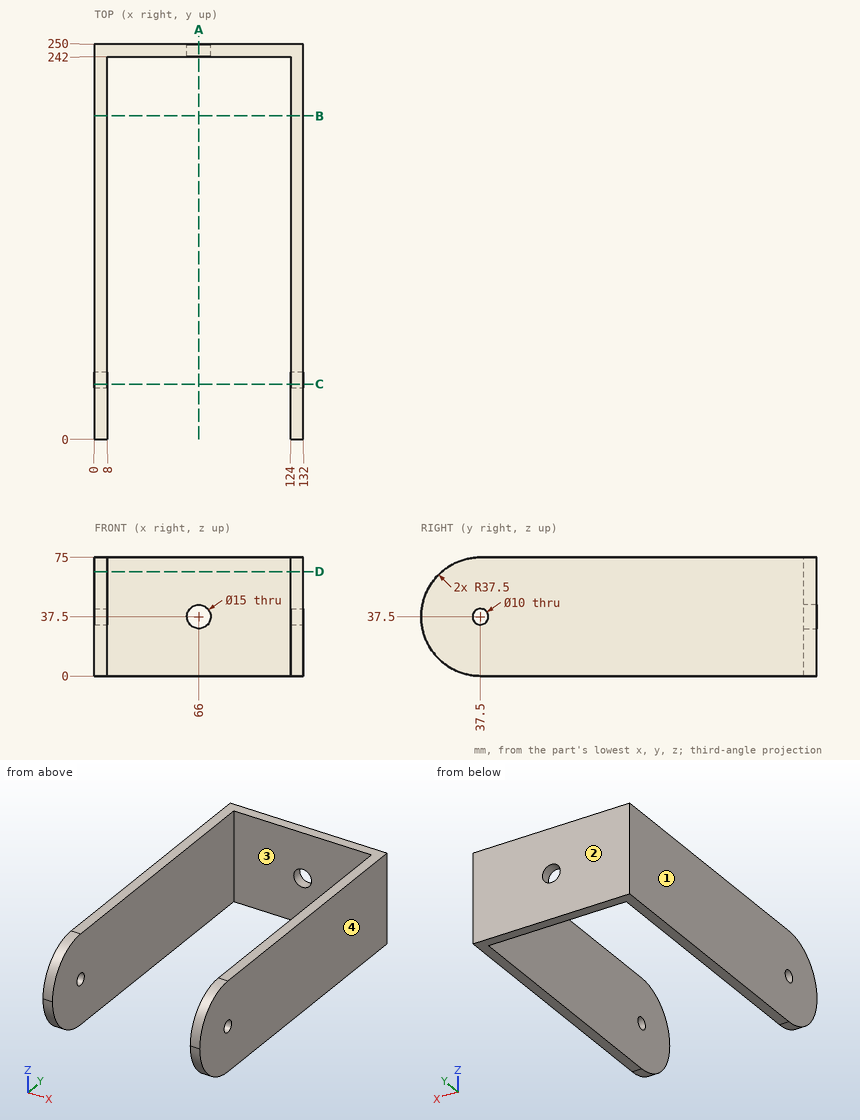
Verification items for this drawing (mm, ordinates from the low corner). Coordinates: 2 decimals unless noted, no trailing zeros. Order: outer loops, then holes, each group sorted by start corner. A loop starts at its lowest first (then second) coordinate and runs counter-clockwise, first axis right, second up. Notation, with made-up numbers: M -15.75,16 L 15.25,16 A20 ccw 15.25,46 Z; hole C 17.5,89.5 d4. An arc over 180 degrees is marked long. Write each question's results on one line, items separated by ' | '.
1) Section check A-A on x = 66. Record the cut outline in (y, z).
Solved:
outline: M 242,0 L 250,0 L 250,30 L 242,30 Z; M 242,45 L 250,45 L 250,75 L 242,75 Z
2) Release check for a two-part mould opening along X. For the marked faces 1, 2, 3 and 4 record: pulls with the +X half, pulls with the -X half, needs draft (parallel to the pull), parting line crosses it, or undercut.
Solved:
face 1: pulls with the -X half | face 2: needs draft | face 3: undercut | face 4: pulls with the +X half
3) Section check B-B on y = 204.5. Record the cut outline in (x, z), plus the area to 3 significant figures.
Solved:
outline: M 0,0 L 8,0 L 8,75 L 0,75 Z; M 124,0 L 132,0 L 132,75 L 124,75 Z | area: 1,200 mm²
4) Gauge pin test, flat ends, axial feed: pin 1 Ø5 at (x, z) = (58.5, 14) entering from -Y; pin 2 Ø6 at (y, z) = (37.5, 37.5) entering from -X. Record the tip position at first contact, or that the pin passes through.
Solved:
pin 1: stops at y = 242 | pin 2: passes through
5) Section check D-D on z = 66. Record the cut outline in (x, y), plus the area to 3 significant figures.
Solved:
outline: M 0,13.13 L 8,13.13 L 8,242 L 124,242 L 124,13.13 L 132,13.13 L 132,250 L 0,250 Z | area: 4,720 mm²
6) Scan lines: line 1 along X through (y, z) = (85, 6); line 2 along X through (y, z) = (245, 37.5); line 3 along Z through (x, y) = (128, 37.5). Record each from-to range of solid material in increasing order. Write a range as [from, to].
Solved:
line 1: x = [0, 8], [124, 132] | line 2: x = [0, 58.5], [73.5, 132] | line 3: z = [0, 32.5], [42.5, 75]
7) Section check C-C on y = 35. Record the cut outline in (x, z), plus the area to 3 significant figures.
Solved:
outline: M 0,0.08 L 8,0.08 L 8,33.17 L 0,33.17 Z; M 0,41.83 L 8,41.83 L 8,74.92 L 0,74.92 Z; M 124,0.08 L 132,0.08 L 132,33.17 L 124,33.17 Z; M 124,41.83 L 132,41.83 L 132,74.92 L 124,74.92 Z | area: 1,060 mm²
